from build123d import *

# Parameters (mm, degrees)
SKETCH1_W           = 15.25
SKETCH1_H           = 48.75
BOSS_EXTRUDE1_DEPTH = 10.5
SHELL1_T            = -0.25
SKETCH3_W           = 6.5
SKETCH3_H           = 10.5
BOSS_EXTRUDE2_DEPTH = 0.5


with BuildPart() as part:
    # Sketch1 → Boss-Extrude1 (new body)
    with BuildSketch(Plane(origin=(0, 0, 0), x_dir=(1, 0, 0), z_dir=(0, 1, 0))):
        with Locations((-7.625, -16.379710312)):
            Rectangle(SKETCH1_W, SKETCH1_H)
    extrude(amount=BOSS_EXTRUDE1_DEPTH)

    # Shell1
    shell1_openings = [part.faces().sort_by_distance(p)[0] for p in [
        (-7.625, 5.25, 40.754710312),
    ]]
    offset(amount=SHELL1_T, openings=shell1_openings, kind=Kind.INTERSECTION)

    # Sketch3 → Boss-Extrude2 (add)
    with BuildSketch(Plane(origin=(0, 0, 0), x_dir=(0, 0, -1), z_dir=(1, 0, 0))):
        with Locations((-36.75, 5.25)):
            Rectangle(SKETCH3_W, SKETCH3_H)
    boss_extrude2 = extrude(amount=BOSS_EXTRUDE2_DEPTH)

    # Mirror1: Boss-Extrude2 across plane
    add(boss_extrude2.mirror(Plane.ZY.offset(7.625)))


solid = part.part
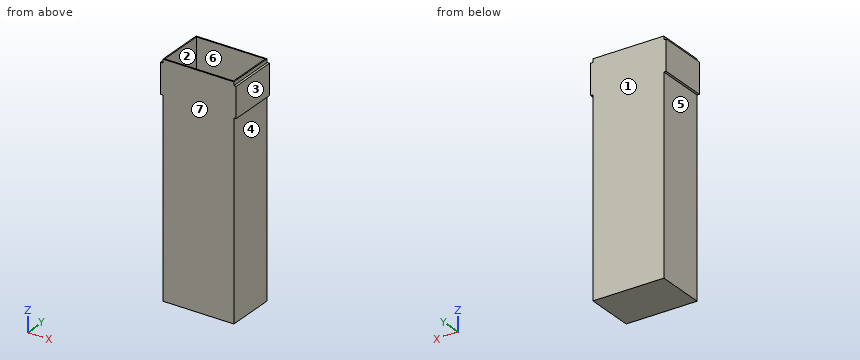
The listing builds one solid part. Answer for the finished solid, in the listing's coordinates (mm). Face numbers are marked on the shaded views. A direction names the side the tool comes from. Coordinates: 2 decimals unless noted, no trailing zeros. Loops run counter-clockwise (first coordinate to the right, second up) from the corner with the lowest first, then second, coordinate; pieces in that order, holes last. Notation, with made-up numbers: (41.5, 63) -> (52.5, 63) arc R16 cw to (52.5, 74) -> close; hole circle Ø9 at (22.5, 76.25). An arc over 180 degrees is marked (long way). Write item = value, one per line. Start each with the question number.
1) The mould has two halves that part along X. Classify the marked faces 1, 2 and 3: released by +X, released by -X, zero draft, split by the parting line, or undercut.
2) A tool of negligible diameter and unlimited length cuts with its end or side. For the marked faces 4, 5, 6 and 7, from which of +Z, -Z, +X, -X, +Y, -Y can it reach the whole face along a straight path? Write none if from no direction.
3) Given pin 1 Ø3 at (y, z) = (6.5, 10) entering from -X; pin 2 Ø2 at (x, z) = (-3.5, 11.5) entering from -Y; pin 3 Ø0.8 at (y, z) = (3, 40.5) entering from +X, each flat-ended and moving along its own axis, determine where each tip first touches the part or whether it passes through.
4) A cutting plane is placed at C-C (y = 2.25). Give the vertices of the cut face in (x, z).
5) A cutting plane is placed at B-B (x = -6.25). Give the vertices of the cut face in (y, z), then the cut area to 3 significant figures.
6) Straight lines are drawn through the part: line 1 (Y direction, x = -14.75, z = 31.5); line 2 (X direction, y = 4.25, z = 20); line 3 (X direction, y = 3, z = 34). For each, find the intervals that lie inside material, in ascending order. Write a range as from..to.
7) A cutting plane is placed at D-D (z = 23). Give the vertices of the cut face in (x, y).
8) A cutting plane is placed at A-A (z = 36). Give the vertices of the cut face in (x, y).
Responses:
q1.face_1 = zero draft
q1.face_2 = undercut
q1.face_3 = released by +X
q2.face_4 = -Z, +X, +Y, -Y
q2.face_5 = -Z, -X, +Y, -Y
q2.face_6 = +Z
q2.face_7 = +Z, -Z, +X, -X, -Y
q3.pin_1 = -15.25
q3.pin_2 = 0
q3.pin_3 = 0
q4.outline = (-15.75, 33.5) -> (-15.25, 33.5) -> (-15.25, -8) -> (0, -8) -> (0, 33.5) -> (0.5, 33.5) -> (0.5, 40) -> (0, 40) -> (0, 40.75) -> (-0.25, 40.75) -> (-0.25, -7.75) -> (-15, -7.75) -> (-15, 40.75) -> (-15.25, 40.75) -> (-15.25, 40) -> (-15.75, 40) -> close
q5.outline = (0, -8) -> (10.5, -8) -> (10.5, 40.75) -> (10.25, 40.75) -> (10.25, -7.75) -> (0.25, -7.75) -> (0.25, 40.75) -> (0, 40.75) -> close
q5.area = 26.9 mm²
q6.line_1 = 0..0.25, 10.25..10.5
q6.line_2 = -15.25..-15, -0.25..0
q6.line_3 = -15.75..-15, -0.25..0.5
q7.outline = (-15.25, 0) -> (0, 0) -> (0, 10.5) -> (-15.25, 10.5) -> close; hole (-15, 0.25) -> (-0.25, 0.25) -> (-0.25, 10.25) -> (-15, 10.25) -> close
q8.outline = (-15.75, 0) -> (0.5, 0) -> (0.5, 10.5) -> (-15.75, 10.5) -> close; hole (-15, 0.25) -> (-0.25, 0.25) -> (-0.25, 10.25) -> (-15, 10.25) -> close
